```python
from build123d import *

# Parameters (mm, degrees)
BOSS_EXTRUDE2_DEPTH                               = 22.225
BOSS_EXTRUDE2_DEPTH_BACK                          = 10
SKETCH2_W                                         = 153.14353988
SKETCH2_H                                         = 6.35
CUT_EXTRUDE1_DEPTH                                = 4.7625
SKETCH3_W                                         = 152.758434582
SKETCH3_H                                         = 6.35
CUT_EXTRUDE2_DEPTH                                = 4.7625
FILLET3_R                                         = 12.7
FILLET4_R                                         = 12.7
FILLET5_R                                         = 12.7
FILLET6_R                                         = 12.7
CUT_EXTRUDE3_DEPTH                                = 94.675
CUT_EXTRUDE3_DEPTH_BACK                           = 84.675
SKETCH12_R                                        = 168.402
CSK_FOR_8_FLAT_HEAD_SOCKET_CAP_SCREW2_D           = 4.4958
CSK_FOR_8_FLAT_HEAD_SOCKET_CAP_SCREW2_CSINK_D     = 9.1186
CSK_FOR_8_FLAT_HEAD_SOCKET_CAP_SCREW2_CSINK_ANGLE = 82
SKETCH24_W                                        = 181.235061551
SKETCH24_H                                        = 69.255288946
CUT_EXTRUDE5_DEPTH                                = 84.675


with BuildPart() as part:
    # Sketch1 → Boss-Extrude2 (new, two sides: drawn at the far end of the back side and taken through both)
    with BuildSketch(Plane(origin=(0, 0, 0), x_dir=(1, 0, 0), z_dir=(0, 1, 0)).offset(-BOSS_EXTRUDE2_DEPTH_BACK)):
        with BuildLine():
            Line((37.204956004, 9.525), (-37.204956004, 9.525))
            ThreePointArc((-37.204956004, 9.525), (-39.498289417, 9.316221792), (-41.716221563, 8.696751473))
            Line((-41.716221563, 8.696751473), (-62.649818949, 0.741984467))
            ThreePointArc((-62.649818949, 0.741984467), (-63.161614851, 0), (-62.649818949, -0.741984467))
            Line((-62.649818949, -0.741984467), (-41.716221563, -8.696751473))
            ThreePointArc((-41.716221563, -8.696751473), (-39.498289417, -9.316221792), (-37.204956004, -9.525))
            Line((-37.204956004, -9.525), (37.204956004, -9.525))
            ThreePointArc((37.204956004, -9.525), (39.498289417, -9.316221792), (41.716221563, -8.696751473))
            Line((41.716221563, -8.696751473), (62.649818949, -0.741984467))
            ThreePointArc((62.649818949, -0.741984467), (63.161614851, 0), (62.649818949, 0.741984467))
            Line((62.649818949, 0.741984467), (41.716221563, 8.696751473))
            ThreePointArc((41.716221563, 8.696751473), (39.498289417, 9.316221792), (37.204956004, 9.525))
        make_face()
    extrude(amount=BOSS_EXTRUDE2_DEPTH + BOSS_EXTRUDE2_DEPTH_BACK)

    # Sketch2 → Cut-Extrude1 (cut)
    with BuildSketch(Plane.XY.offset(9.525)):
        with Locations((7.894658594, 12.7)):
            Rectangle(SKETCH2_W, SKETCH2_H)
    extrude(amount=-CUT_EXTRUDE1_DEPTH, mode=Mode.SUBTRACT)

    # Sketch3 → Cut-Extrude2 (cut)
    with BuildSketch(Plane(origin=(0, 0, -9.525), x_dir=(-1, 0, 0), z_dir=(0, 0, -1))):
        with Locations((8.600684972, 12.7)):
            Rectangle(SKETCH3_W, SKETCH3_H)
    extrude(amount=-CUT_EXTRUDE2_DEPTH, mode=Mode.SUBTRACT)

    # Fillet3
    fillet3_edges = [part.edges().sort_by_distance(p)[0] for p in [
        (52.069514915, 12.7, -4.7625),
    ]]
    fillet(fillet3_edges, radius=FILLET3_R)

    # Fillet4
    fillet4_edges = [part.edges().sort_by_distance(p)[0] for p in [
        (52.069514915, 12.7, 4.7625),
    ]]
    fillet(fillet4_edges, radius=FILLET4_R)

    # Fillet5
    fillet5_edges = [part.edges().sort_by_distance(p)[0] for p in [
        (-52.069514915, 12.7, 4.7625),
    ]]
    fillet(fillet5_edges, radius=FILLET5_R)

    # Fillet6
    fillet6_edges = [part.edges().sort_by_distance(p)[0] for p in [
        (-52.069514915, 12.7, -4.7625),
    ]]
    fillet(fillet6_edges, radius=FILLET6_R)

    # Sketch12 → Cut-Extrude3 (cut, two sides: drawn at the far end of the back side and taken through both)
    with BuildSketch(Plane(origin=(0, 0, 0), x_dir=(0, 0, -1), z_dir=(1, 0, 0)).offset(-CUT_EXTRUDE3_DEPTH_BACK)):
        with Locations((0, -168.402)):
            Circle(SKETCH12_R)
    extrude(amount=CUT_EXTRUDE3_DEPTH + CUT_EXTRUDE3_DEPTH_BACK, mode=Mode.SUBTRACT)

    # CSK for #8 Flat Head Socket Cap Screw2 (through all)
    with Locations(Plane(origin=(0, 22.225, 0), x_dir=(1, 0, 0), z_dir=(0, 1, 0))):
        with Locations((-44.45, 0), (44.45, 0)):
            CounterSinkHole(CSK_FOR_8_FLAT_HEAD_SOCKET_CAP_SCREW2_D / 2, CSK_FOR_8_FLAT_HEAD_SOCKET_CAP_SCREW2_CSINK_D / 2, counter_sink_angle=CSK_FOR_8_FLAT_HEAD_SOCKET_CAP_SCREW2_CSINK_ANGLE)

    # Sketch24 → Cut-Extrude5 (cut)
    with BuildSketch(Plane(origin=(0, 15.875, 0), x_dir=(1, 0, 0), z_dir=(0, 1, 0))):
        with Locations((3.936847216, -3.169453317)):
            Rectangle(SKETCH24_W, SKETCH24_H)
    extrude(amount=-CUT_EXTRUDE5_DEPTH, mode=Mode.SUBTRACT)


solid = part.part
```
Can you work these out from the model? Positions are in its coordinate system, mm. Coordinates: 2 decimals unless noted, no trailing zeros. Loops run counter-clockwise (first coordinate to the right, second up) from the corner with the lowest first, then second, coordinate; pieces in that order, holes last. Notation, with made-up numbers: (52.25, 28.5) -> (77.25, 28.5) arc R19 cw to (77.25, 52.5) -> close; hole circle Ø11 at (1.25, 17.25). An arc over 180 degrees is marked (long way). Put each result on its own line as item: value. Start each with the question number.
Q1. Thinking about a two-plate mould opening in X: for faces 1 (the face through (-42.67, 17.69, 1.37)), 2 (the face through (-52.33, 19.006, 4.664)), 3 (the face through (-1, 19, 9.525)), 4 (the face through (-42.577, 19.695, 1.436)), which applies, pulls with the +X half, pulls with the -X half, needs draft (parallel to the pull), parting line crosses it, or undercut?
Q2. I want a section at A-A (y = 18.5). Count the separate pieces of the cut face and the enclosed holes in it, plus the area to 3 significant figures.
Q3. If I drill on line 1 (Z direction, x = 44.45, y = 16.9); line 2 (Z direction, x = 45.5, y = 16.5); line 3 (Y direction, x = -41, z = -1.75) (3 decimals), over which ranges is the centre line in solid material (lowest first)? Write a range as [from, to].
Q4. I'm going to push a flat-ended pin straight in: P1, Ø3, axis at x = 43.5, y = 20, coming from the +Z side. Where does the tip first touch, or does it pass through?
Q5. I want a section at B-B (x = -44.45). Write out the boundary of the cut face in (y, z) (3 decimals).
Taken from the geometry:
1. face 1: undercut
1. face 2: pulls with the -X half
1. face 3: needs draft
1. face 4: undercut
2. separate pieces: 1
2. enclosed holes: 2
2. area: 1,950 mm2
3. line 1: z = [-7.66, -2.25], [2.25, 7.66]
3. line 2: z = [-7.26, -1.99], [1.99, 7.26]
3. line 3: y = [15.875, 21.43]
4. P1: stops at z = 8.59
5. outline: (15.875, -7.658) -> (22.225, -7.658) -> (22.225, -4.559) -> (19.566, -2.248) -> (15.875, -2.248) -> close; (15.875, 2.248) -> (19.566, 2.248) -> (22.225, 4.559) -> (22.225, 7.658) -> (15.875, 7.658) -> close
